Here's how the part is built. I have some questions about the finished solid (model axes, mm). Face numbers are marked on the shaded views. Coordinates: 2 decimals unless noted, no trailing zeros. Order: outer loops, then holes, each group sorted by start corner. A loop starts at its lowest first (then second) coordinate and runs counter-clockwise, first axis right, second up. Notation, with made-up numbers: (-27, 80) - (-3, 80) arc R14 ccw to (-3, 107) - close; hole circle Ø7 at (-3, 9). An arc over 180 degrees is marked (long way). Answer in a Markdown table with one row per item. Add a question column.
Item 1: I want a section at C-C (z = -40). Please give me the cut outline in (x, y).
Item 2: I want a section at A-A (x = 32.5). Please give me the cut outline in (y, z).
Item 3: I want a section at D-D (x = -27.5). Please give me the cut outline in (y, z), plus the area to 4 significant figures.
Item 4: I want a section at B-B (y = -3.25). Please give me the cut outline in (x, z).
Item 5: Thinking about a two-plate mould opening in Y: for the marked faces 1 and 2, which applies, +Y half, -Y half, draft (parallel to the pull), parting line (faces both ways), or undercut?
Item 6: Will these pins go through, and if not, where does the flat tip stop? pin 1 Ø7.5 at (x, z) = (32.5, -40) entering from -Y; pin 2 Ø12 at (x, z) = (12, 19.5) entering from +Y; pin 3 Ø4 at (y, z) = (-5, 38) entering from -X; pin 4 Ø4 at (x, y) = (-16, -2.5) entering from +Z.
Item 7: If I drill on line 1 along Z through (x, y) = (-27.5, -4); line 2 along Z through (x, y) = (32.5, -2.5); line 3 along Z through (x, y) = (35.5, -1.5), over which ranges is the centre line in solid material (lowest first)? Write a range as from..to.
```python
from build123d import *

# Parameters (mm, degrees)
F0_W     = 95
F0_H     = 105
F0_R     = 4.25
F1_DEPTH = 8
F2_SIZE  = 0.5
F3_W     = 50
F3_H     = 55.8646805584
F4_DEPTH = 25


with BuildPart() as f1:
    # F0 (on Front) → F1 (new body)
    with BuildSketch(Plane.XZ):
        with Locations((2.5, 0)):
            Rectangle(F0_W, F0_H)
        with Locations((-27.5, -40)):
            Circle(F0_R, mode=Mode.SUBTRACT)
        with Locations((32.5, -40)):
            Circle(F0_R, mode=Mode.SUBTRACT)
        with Locations((-27.5, 0)):
            Circle(F0_R, mode=Mode.SUBTRACT)
        with Locations((32.5, 0)):
            Circle(F0_R, mode=Mode.SUBTRACT)
        with Locations((32.5, 40)):
            Circle(F0_R, mode=Mode.SUBTRACT)
    extrude(amount=F1_DEPTH)

    # F2
    f2_edges = [f1.edges().sort_by_distance(p)[0] for p in [
        (28.25, -8, 40),
        (28.25, -8, -40),
        (-31.75, -8, -40),
        (-31.75, -8, 0),
        (28.25, -8, 0),
    ]]
    chamfer(f2_edges, length=F2_SIZE)

    # F3 (on face) → F4 (cut)
    with BuildSketch(Plane.XZ.offset(8)):
        with Locations((-30, 60.4323402792)):
            Rectangle(F3_W, F3_H)
    extrude(amount=-F4_DEPTH, mode=Mode.SUBTRACT)


solid = f1.part
```
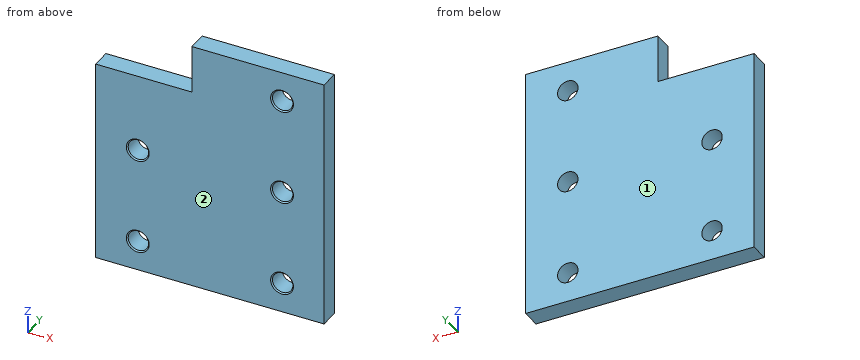
Values follow:
| question | item | result |
|---|---|---|
| 1 | outline | (-45, -8) - (-32.25, -8) - (-31.75, -7.5) - (-31.75, 0) - (-45, 0) - close; (-23.25, -7.5) - (-22.75, -8) - (27.75, -8) - (28.25, -7.5) - (28.25, 0) - (-23.25, 0) - close; (36.75, -7.5) - (37.25, -8) - (50, -8) - (50, 0) - (36.75, 0) - close |
| 2 | outline | (-8, -52.5) - (0, -52.5) - (0, -44.25) - (-7.5, -44.25) - (-8, -44.75) - close; (-8, -35.25) - (-7.5, -35.75) - (0, -35.75) - (0, -4.25) - (-7.5, -4.25) - (-8, -4.75) - close; (-8, 4.75) - (-7.5, 4.25) - (0, 4.25) - (0, 35.75) - (-7.5, 35.75) - (-8, 35.25) - close; (-8, 44.75) - (-7.5, 44.25) - (0, 44.25) - (0, 52.5) - (-8, 52.5) - close |
| 3 | outline | (-8, -52.5) - (0, -52.5) - (0, -44.25) - (-7.5, -44.25) - (-8, -44.75) - close; (-8, -35.25) - (-7.5, -35.75) - (0, -35.75) - (0, -4.25) - (-7.5, -4.25) - (-8, -4.75) - close; (-8, 4.75) - (-7.5, 4.25) - (0, 4.25) - (0, 32.5) - (-8, 32.5) - close |
| 3 | area | 543.5 mm^2 |
| 4 | outline | (-45, -52.5) - (50, -52.5) - (50, 52.5) - (-5, 52.5) - (-5, 32.5) - (-45, 32.5) - close; hole circle Ø8.5 at (-27.5, -40); hole circle Ø8.5 at (-27.5, 0); hole circle Ø8.5 at (32.5, -40); hole circle Ø8.5 at (32.5, 0); hole circle Ø8.5 at (32.5, 40) |
| 5 | face 1 | +Y half |
| 5 | face 2 | -Y half |
| 6 | pin 1 | passes through |
| 6 | pin 2 | stops at y = 0 |
| 6 | pin 3 | stops at x = -5 |
| 6 | pin 4 | stops at z = 32.5 |
| 7 | line 1 | z = -52.5..-44.25, -35.75..-4.25, 4.25..32.5 |
| 7 | line 2 | z = -52.5..-44.25, -35.75..-4.25, 4.25..35.75, 44.25..52.5 |
| 7 | line 3 | z = -52.5..-43.01, -36.99..-3.01, 3.01..36.99, 43.01..52.5 |
